Input: part model. Units: mm. Frame: model coordinates. Face numbers are marked on the shaded views. Coordinates: 2 decimals unless noted, no trailing zeros. Write each loop counter-clockwise with the first axis right and the second up, starting at its lowest first coordinate (ties: lowest second). Pieces come first, ordered by that corner, then holes. Notation, with made-up numbers: (-27, -25) - (12, -25) arc R31 ccw to (12, 2) - close; hole circle Ø11 at (8, 68.25). An arc over 180 degrees is marked (long way). Use a Markdown table: item, result. Add a question column.
Q1. Pin query (flat end, axial travel): P1, Ø1, axis at y = 51, z = -2.5, coming from the -X side; P2, Ø3, axis at x = 0, z = 0, coming from the -Y side; P3, Ø5.5, axis at x = 0.5, z = 0, coming from the -Y side; P4, Ø6, axis at y = 15.5, z = 5, coming from the +X side. Return the tip coordinate at first contact, or that it passes through.
Q2. Section query D-D (z = 4.5). Return the cut outline in (x, y).
Q3. Mould query, pull axis X, two halves, no side actions, for the marked faces 1, 2, 3 and 4. Classes: released by +X, released by -X, zero draft, split by the parting line, or undercut.
Q4. Section query B-B (x = 0). Return the cut outline in (y, z), then the cut area to 3 significant figures.
Q5. Material intervals for probe 1 along Z at (x, y) = (0, 74.25); probe 2 along X at (y, z) = (74, 0); probe 3 along Y at (x, z) = (-2, 1.5), sorted ascending. Write a range as from..to.
Q6. Section query A-A (y = 78). Return the cut outline in (x, z).
Q7. Section query C-C (y = 37). Return the cut outline in (x, z).
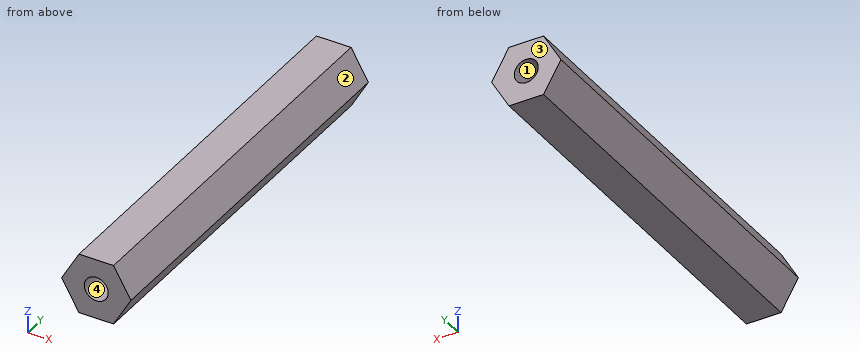
Autodesk Inventor part; units mm, degrees
ref_plane "YZ Plane" through (0, 0, 0) normal (1, 0, 0) x (0, 1, 0)
ref_plane "XZ Plane" through (0, 0, 0) normal (0, 1, 0) x (-1, 0, 0)
ref_plane "XY Plane" through (0, 0, 0) normal (0, 0, 1) x (1, 0, 0)
sketch "Sketch1" plane through (0, 0, 0) normal (0, 1, 0) x (-1, 0, 0)
  line L0 (-3.6662, 6.35) -> (3.6662, 6.35)
  line L1 (3.6662, 6.35) -> (7.3323, 0)
  line L2 (7.3323, 0) -> (3.6662, -6.35)
  line L3 (3.6662, -6.35) -> (-3.6662, -6.35)
  line L4 (-3.6662, -6.35) -> (-7.3323, 0)
  line L5 (-7.3323, 0) -> (-3.6662, 6.35)
  point P0 (0, 0)
  point P1 (0, 0)
  dimension "d0" = 12.7
extrude "Extrusion1" add sketch "Sketch1" along normal blind 84.0867
sketch "Sketch2" plane through (0, 84.0867, 0) normal (0, 1, 0) x (1, 0, 0)
  circle A0 centre (0, 0) radius 2.54
  dimension "d3" = 5.08
extrude "Extrusion2" cut sketch "Sketch2" against normal blind 25.4
thread "Thread1"
sketch "Sketch3" plane through (0, 0, 0) normal (0, -1, 0) x (1, 0, 0)
  circle A0 centre (0, 0) radius 2.54
  dimension "d8" = 5.08
extrude "Extrusion3" cut sketch "Sketch3" against normal blind 25.4
thread "Thread2"
properties part number "OUTK_015_Shaft2" material "Aluminum 6061"
Values follow:
| question | item | result |
|---|---|---|
| 1 | P1 | x = -6.18 |
| 1 | P2 | y = 25.4 |
| 1 | P3 | y = 0 |
| 1 | P4 | x = 6.18 |
| 2 | outline | (-4.73, 0) - (4.73, 0) - (4.73, 84.09) - (-4.73, 84.09) - close |
| 3 | face 1 | undercut |
| 3 | face 2 | released by +X |
| 3 | face 3 | zero draft |
| 3 | face 4 | undercut |
| 4 | outline | (0, -6.35) - (84.09, -6.35) - (84.09, -2.54) - (58.69, -2.54) - (58.69, 2.54) - (84.09, 2.54) - (84.09, 6.35) - (0, 6.35) - (0, 2.54) - (25.4, 2.54) - (25.4, -2.54) - (0, -2.54) - close |
| 4 | area | 810 mm2 |
| 5 | probe 1 | -6.35..-2.54, 2.54..6.35 |
| 5 | probe 2 | -7.33..-2.54, 2.54..7.33 |
| 5 | probe 3 | 25.4..58.69 |
| 6 | outline | (-7.33, 0) - (-3.67, -6.35) - (3.67, -6.35) - (7.33, 0) - (3.67, 6.35) - (-3.67, 6.35) - close; hole circle Ø5.08 at (0, 0) |
| 7 | outline | (-7.33, 0) - (-3.67, -6.35) - (3.67, -6.35) - (7.33, 0) - (3.67, 6.35) - (-3.67, 6.35) - close |
